Could you check a few things on this model? Use its own coordinates, in mm. Face numbers are marked on the shaded views. A direction names the side the tool comes from. Round coordinates to 2 decimals unless told otherwise and drop trailing zeros. Order: outer loops, then holes, each group sorted by start corner. A loop starts at its lowest first (then second) coordinate and runs counter-clockwise, first axis right, second up. Notation, with made-up numbers: (9, 22.5) - (48, 22.5) arc R32 ccw to (48, 58.5) - close; hole circle Ø10 at (28.25, -33.5). An arc over 180 degrees is marked (long way). Return JSON: item names as keys, results as strings. Group by question number.
from build123d import *

# Parameters (mm, degrees)
F1_DEPTH = 10
F2_T     = 1
F3_R     = 3.2218950318
F4_DEPTH = 25.4
F5_R     = 5.0145008795
F6_DEPTH = 25.4
F7_W     = 2.708992688
F7_H     = 32.9594105715
F8_DEPTH = 25


with BuildPart() as f1:
    # F0 (on Top) → F1 (new body)
    with BuildSketch(Plane.XY):
        Polygon((-7.9906535461, 28.9775509901), (-5.7124293756, 28.7289765854), (-2.177747665, 18.313806504), (-2.177747665, 15.5732491985), (-3.5480263177, 10.3661902249), (-3.5480263177, 4.4739907607), (-2.177747665, 0), (-3.410998499, -10.1879928261), (-2.177747665, -15.8061366528), (0, -26.4196246862), (0, -29.9038495868), (0, -32.9525433481), (-4.7522801906, -36.7271192372), (-4.846881947, -37.3447827538), (-4.7036297619, -37.9973761737), (-4.3055904098, -38.4158245646), (-3.8245406306, -38.5066020873), (-3.410998499, -38.4158245646), (0, -37.6670689483), (3.2324001659, -35.4205369949), (5.8037610725, -33.2740206294), (5.2963984199, -32.5517579913), (3.7367703403, -30.6914262474), (3.7367703403, -30.091624707), (3.7367703403, -28.8444478065), (3.7367703403, -22.7698273957), (3.7367703403, -15.2410743758), (3.7367703403, -5.9498115443), (5.555216223, -2.1752356552), (5.0777255662, 0), (4.3131460861, 3.4830850037), (3.2794470092, 8.1921595303), (5.119686015, 14.2296506092), (4.5323909172, 16.9051065964), (7.0069744252, 20.4722173512), (6.4797433326, 22.8740483706), (5.119686015, 24.0607738481), (2.6262372261, 23.513431542), (1.6395514831, 21.6216556728), (0, 21.2617542006), (-2.8885214715, 29.960425262), (-2.3250187241, 30.496619276), (-1.3758151717, 31.9517953008), (-0.9570455703, 33.4362002962), (-0.9286604067, 34.6111891241), (-1.1501351436, 35.753425343), (-1.8199630103, 37.1648714688), (-2.8861434893, 38.3458743138), (-4.2181453118, 39.1544558587), (-5.6038486027, 39.5364638273), (-7.0804168612, 39.5364638273), (-8.9181209402, 38.937315781), (-10.336358338, 37.8366215939), (-11.4427582769, 36.0244784539), (-11.7720668322, 34.3284905467), (-11.6132239292, 32.8387650441), (-10.9819831447, 31.3281121322), (-9.9742822169, 30.1140705775), align=None)
    extrude(amount=F1_DEPTH)

    # F2
    f2_openings = [f1.faces().sort_by_distance(p)[0] for p in [
        (-0.518875, 3.902711, 10),
    ]]
    offset(amount=F2_T, openings=f2_openings, kind=Kind.INTERSECTION)

    # F3 (on Top) → F4 (cut)
    with BuildSketch(Plane.XY):
        with Locations((0, 7.7414768748)):
            Circle(F3_R)
    extrude(amount=-F4_DEPTH, mode=Mode.SUBTRACT)

    # F5 (on Top) → F6 (cut)
    with BuildSketch(Plane.XY):
        with Locations((-6.3707926311, 34.1742038727)):
            Circle(F5_R)
    extrude(amount=-F6_DEPTH, mode=Mode.SUBTRACT)

    # F7 (on Top) → F8 (cut)
    with BuildSketch(Plane.XY):
        with Locations((1.9566247938, -18.3495350066)):
            Rectangle(F7_W, F7_H)
    extrude(amount=-F8_DEPTH, mode=Mode.SUBTRACT)


solid = f1.part
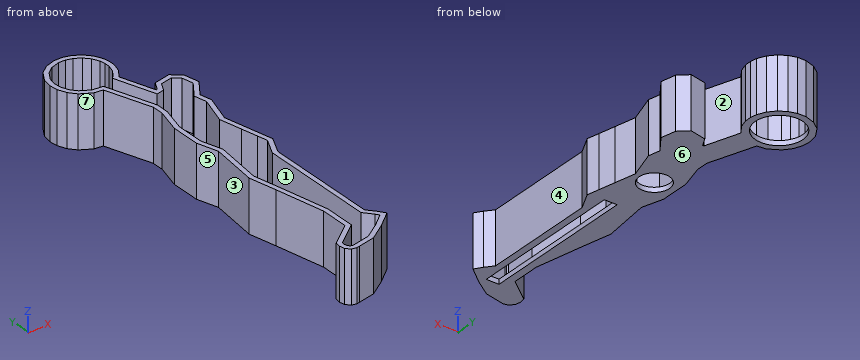
1) I want a section at A-A, the plane y = -8.5. List the corners of the cut face in (x, z) for me, plus the area to 3 significant figures.
2) Will these pins go through, and if not, where does the flat tip stop? pin 1 (5 mm diameter, centred on y = -9, z = 7, fed in from +X); pin 2 (2 mm diameter, centred on x = 0.5, y = -7.5, fed in from +Z); pin 3 (2 mm diameter, centred on x = 5.5, z = 2, fed in from +Y).
3) I want a section at B-B, the plane y = -23.5. List the corners of the cut face in (x, z) for me, plus the area to 3 significant figures.
4) For the marked faces 1, 2, 3 and 4, which set-ups out of +Z, -Z, +X, -X, +Y, -Y let a thin tool reach every point of the face, with its end or its side?
5) If I drill on line 1 along X through (y, z) = (-35, 5.75); line 2 along Y through (x, z) = (-8.75, 6.5); line 3 along X through (y, z) = (16, 7), over which ranges is the centre line in solid material (lowest first)? Write a range as from..to.
6) We'd pull the mould along Y, two halves only. Please class the marked faces 5, 6 and 7: +Y half, -Y half, draft (parallel to the pull), parting line (faces both ways), or undercut.
Outcome:
{
 "1": {"outline": "(-4.21, -1) - (0.6, -1) - (0.6, 0) - (-3.21, 0) - (-3.21, 10) - (-4.21, 10) - close; (3.31, -1) - (4.74, -1) - (4.74, 10) - (3.74, 10) - (3.74, 0) - (3.31, 0) - close", "area": "26.3 mm^2"},
 "2": {"pin 1": "x = 4.74", "pin 2": "z = 0", "pin 3": "y = 25.15"},
 "3": {"outline": "(-1.62, -1) - (0.6, -1) - (0.6, 0) - (-0.6, 0) - (-0.6, 10) - (-1.62, 10) - close; (3.31, -1) - (4.74, -1) - (4.74, 10) - (3.74, 10) - (3.74, 0) - (3.31, 0) - close", "area": "23.9 mm^2"},
 "4": {"face 1": "+Z", "face 2": "+Z, -Z", "face 3": "+Z, -Z, -X", "face 4": "+Z, -Z, +X"},
 "5": {"line 1": "-4.19..-2.58, 3.74..5.3", "line 2": "28.26..29.41, 38.99..40.04", "line 3": "-3.18..-2.18, 4.73..5.75"},
 "6": {"face 5": "undercut", "face 6": "draft", "face 7": "-Y half"}
}
